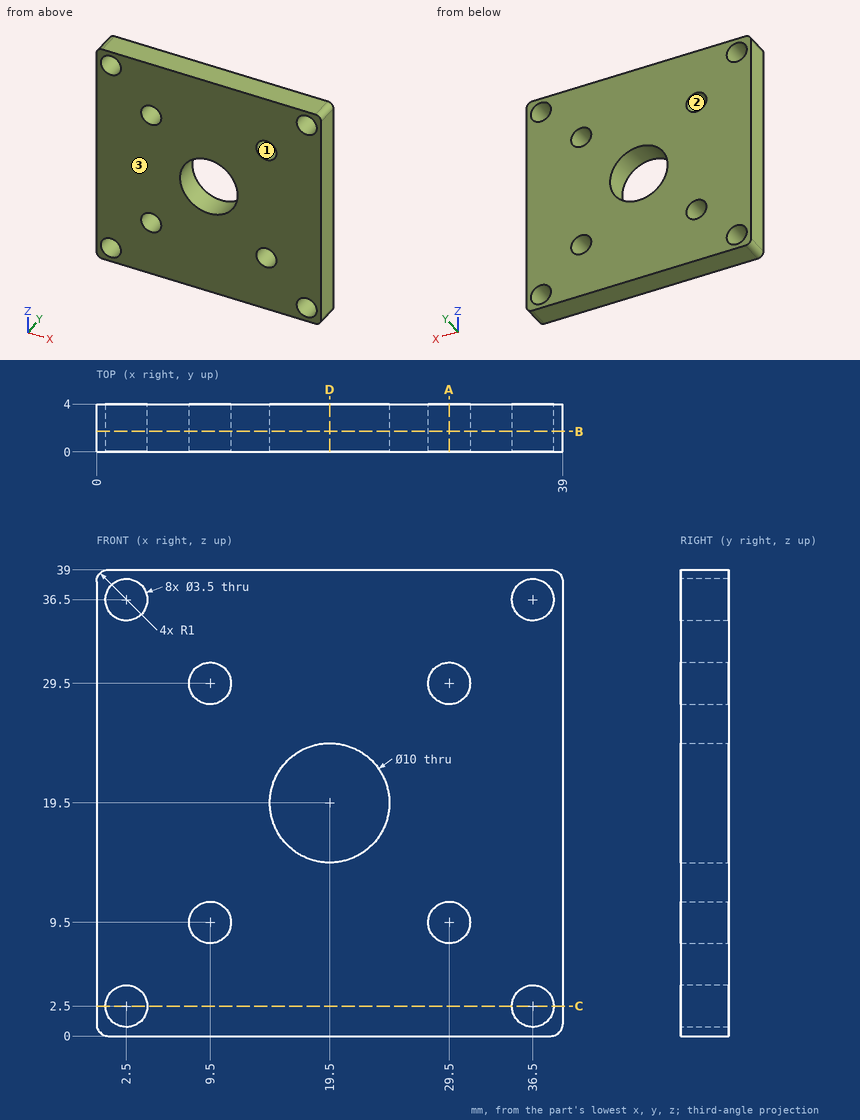
Geometry check sheet. Reference: drawing and pictorial views, mm from the part's lowest x, y, z. Round coordinates to 2 decimals unless told otherwise and drop trailing zeros. Loops run counter-clockwise (first coordinate to the right, second up) from the corner with the lowest first, then second, coordinate; pieces in that order, holes last. Notation, with made-up numbers: (-10.5, -14.5) - (25.5, -14.5) arc R15 cw to (25.5, 9.5) - close; hole circle Ø9 at (54, -20.75). An arc over 180 degrees is marked (long way). Answer as CSV lines item,"result".
(1) Cross-section at D-D, the plane x = 19.5. Enter the section's corners in (y, z), and give its area (3 significant figures).
Output values:
outline,"(0, 0) - (4, 0) - (4, 14.5) - (0, 14.5) - close; (0, 24.5) - (4, 24.5) - (4, 39) - (0, 39) - close"
area,"116 mm²"
(2) Cross-section at B-B, the plane y = 1.7. Give the number of separate pieces and of enclosed holes in the cut face, and give its area (3 significant figures).
Output values:
separate pieces,"1"
enclosed holes,"9"
area,"1,360 mm²"
(3) Cross-section at C-C, the plane z = 2.5. Enter the section's corners in (x, y).
Output values:
outline,"(0, 0) - (0.75, 0) - (0.75, 4) - (0, 4) - close; (4.25, 0) - (34.75, 0) - (34.75, 4) - (4.25, 4) - close; (38.25, 0) - (39, 0) - (39, 4) - (38.25, 4) - close"
(4) Material ranges on line 1 along Z through (x, y) = (2.5, 2.45); line 2 along Z through (x, y) = (9.5, 0.85), recorded low to high.
Output values:
line 1,"z = 0 to 0.75, 4.25 to 34.75, 38.25 to 39"
line 2,"z = 0 to 7.75, 11.25 to 27.75, 31.25 to 39"
(5) Cross-section at A-A, the plane x = 29.5. Enter the section's corners in (y, z).
Output values:
outline,"(0, 0) - (4, 0) - (4, 7.75) - (0, 7.75) - close; (0, 11.25) - (4, 11.25) - (4, 27.75) - (0, 27.75) - close; (0, 31.25) - (4, 31.25) - (4, 39) - (0, 39) - close"
(6) Depth check by flat-ended pin: pin 1 Ø1.5 at (x, y) = (29, 1.5) entering from -Z. Enter the tip coordinate at first touch or a pass-through.
Output values:
pin 1,"stops at z = 0"
(7) Release check for a two-part mould opening along X. For the marked faces 1, 2 and 3 record: released by +X, released by -X, zero draft, split by the parting line, or undercut.
Output values:
face 1,"undercut"
face 2,"undercut"
face 3,"zero draft"
